from build123d import *

# Parameters (mm, degrees)
BOSS_EXTRUDE1_START     = -3
BOSS_EXTRUDE1_DEPTH     = 3
BOSS_EXTRUDE2_DEPTH     = 12
CUT_EXTRUDE1_DEPTH      = 498.153256686
CUT_EXTRUDE1_DEPTH_BACK = 498.153256686
SKETCH4_R               = 2
SKETCH4_R_2             = 2.5


# Read off the part's stored shape, not the designer's step: Boss-Extrude1
with BuildPart() as part:
    # Boss-Extrude1 outline → Boss-Extrude1 (new body)
    with BuildSketch(Plane(origin=(0, 0, 0), x_dir=(0, 0, -1), z_dir=(1, 0, 0)).offset(BOSS_EXTRUDE1_START)):
        with BuildLine():
            Line((374.921925096, 326.088635526), (24.921925096, 326.088635526))
            add(Edge.make_bspline(
                [(24.921925096, 326.088635526), (-144.675070379, 326.088635526), (-139.84656943, 326.088635526), (-375.078074904, 276.088635526)],
                knots=[0, 0, 0, 0, 1, 1, 1, 1], degree=3))
            Line((-375.078074904, 276.088635526), (-375.078074904, -323.911364474))
            add(Edge.make_bspline(
                [(-375.078074904, -323.911364474), (-95.541085852, -323.911364474), (-35.062480537, -311.056240074), (157.348776273, -270.157964899)],
                knots=[0, 0, 0, 0, 1, 1, 1, 1], degree=3))
            Line((157.348776273, -270.157964899), (374.921925096, -223.911364474))
            Line((374.921925096, -223.911364474), (374.921925096, 326.088635526))
        make_face()
    extrude(amount=BOSS_EXTRUDE1_DEPTH)

    # Sketch3 → Boss-Extrude2 (add)
    with BuildSketch(Plane(origin=(0, 0, 0), x_dir=(0, 0, -1), z_dir=(1, 0, 0))):
        Polygon((157.348776273, -270.157964899), (374.921925096, -223.911364474), (374.921925096, 326.088635526), (371.921925096, 326.088635526), (371.921925096, -221.482012374), (156.725041201, -267.223522097), align=None)
    extrude(amount=BOSS_EXTRUDE2_DEPTH)

    # Sketch4 → Cut-Extrude1 (cut, two sides: drawn at the far end of the back side and taken through both)
    with BuildSketch(Plane(origin=(0, 0, 0), x_dir=(0, 0, -1), z_dir=(1, 0, 0)).offset(-CUT_EXTRUDE1_DEPTH_BACK)):
        with Locations((25.083553444, -44.01739539)):
            Circle(SKETCH4_R)
        with Locations((357.01536917, 269.230000887)):
            Circle(SKETCH4_R)
        with Locations((344.332369965, 247.678292183)):
            Circle(SKETCH4_R)
        with Locations((309.057260956, 151.668432327)):
            Circle(SKETCH4_R_2)
        with Locations((258.591204121, 110.126241652)):
            Circle(SKETCH4_R_2)
        with Locations((-61.91870145, 282.615467423)):
            Circle(SKETCH4_R)
        with Locations((-84.669558452, 272.236010663)):
            Circle(SKETCH4_R)
        with Locations((-175.680236141, 229.281564523)):
            Circle(SKETCH4_R_2)
        with Locations((-240.980976375, 232.178083695)):
            Circle(SKETCH4_R_2)
        with Locations((-139.344950951, -53.676954932)):
            Circle(SKETCH4_R)
    extrude(amount=CUT_EXTRUDE1_DEPTH + CUT_EXTRUDE1_DEPTH_BACK, mode=Mode.SUBTRACT)


solid = part.part
Can you work these out from the model? Positions are in its coordinate system, mm. A direction names the side the tool comes from. Coordinates: 2 decimals unless noted, no trailing zeros. Order: outer loops, then holes, each group sorted by start corner. A loop starts at its lowest first (then second) coordinate and runs counter-clockwise, first axis right, second up. Notation, with made-up numbers: (-37, 53) - (-26, 53) arc R12 ccw to (-26, 74) - close; hole circle Ø3 at (-20, -15). An arc over 180 degrees is marked (long way). Answer as a JSON object with one key per item and string values. Group by question number.
Q1. On a 3-axis mill with a long thin cutter (end or side, diameter ignored), from which of +Z, -Z, +X, -X, +Y, -Y can I reach the whole of each face in a straight line? I mean faces 1 (the face through (-2, 326.089, -201)), 2 (the face through (0, 6, 7)). Say none if no direction works.
Q2. I need wall thicknesses on line 1 (X direction, y = 300.5, z = 227); line 2 (Z direction, x = 0.75, y = -18); line 3 (Y direction, x = 3.5, z = -312). Which ranges of each line are inside material? Lowest first, please. Write a range as from..to.
Q3. Imagine slicing it at B-B (z = -202). Please give me the cut outline in (x, y), and give its area (3 significant figures).
Q4. Will these pins go through, and if not, where does the flat tip stop? P1, Ø6, axis at y = 110.13, z = -258.59, coming from the +X side; P2, Ø8, axis at x = 3.5, z = 152, coming from the +Y side; P3, Ø3.5, axis at x = 8, y = -25, coming from the +Z side.
Q5. Imagine slicing it at A-A (x = 3.25). Please give me the cut outline in (y, z).
Determined:
{
 "1": {"face 1": "+Z, -Z, +X, -X, +Y", "face 2": "+Z, +X, +Y"},
 "2": {"line 1": "x = -3..0", "line 2": "z = -374.92..-371.92", "line 3": "y = -237.29..-234.22"},
 "3": {"outline": "(-3, -260.67) - (12, -260.67) - (12, -257.6) - (0, -257.6) - (0, 326.09) - (-3, 326.09) - close", "area": "1,800 mm2"},
 "4": {"P1": "stops at x = 0", "P2": "stops at y = 319.89", "P3": "stops at z = -371.92"},
 "5": {"outline": "(-270.16, -157.35) - (-223.91, -374.92) - (326.09, -374.92) - (326.09, -371.92) - (-221.48, -371.92) - (-267.22, -156.73) - close"}
}
